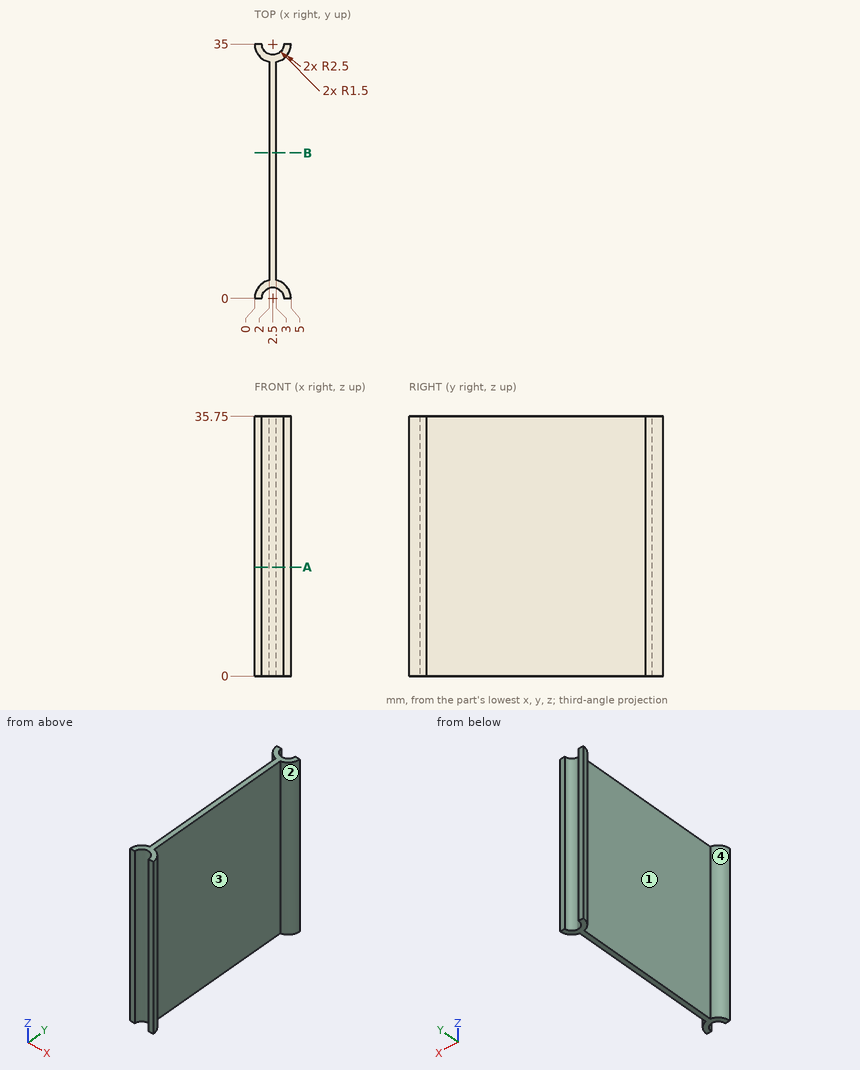
For this review, use the dimensioned drawing (mm, ordinates from the lowest corner) and the shaded views. A direction names the side the tool comes from. Round coordinates to 2 decimals unless told otherwise and drop trailing zeros. Order: outer loops, then holes, each group sorted by start corner. A loop starts at its lowest first (then second) coordinate and runs counter-clockwise, first axis right, second up. Notation, with made-up numbers: M -2.75,-7 L 33.25,-7 A12 cw 33.25,3 Z; hole C -12.75,46.5 d10. An arc over 180 degrees is marked long. Use a Markdown table: item, result. Add a question column.
Item 1: Add section B-B, the plane y = 20. Give the boundary of the cut face in (x, z), then the cut area to 4 significant figures.
Item 2: Insertion check: pin 1 (1.5 mm diameter, centred on x = 1, y = 12, fed in from -Z); pin 2 (3 mm diameter, centred on x = 3, z = 26.5, fed in from +Y); pin 3 (9 mm diameter, centred on y = 23, z = 12.5, fed in from -X). Each pin has a flat end and moves straight along its axis. Give the tip position at first contact, or say it passes through.
Item 3: Mouldability with a two-part tool opening along Y and no side actions: class the marked faces 3 and 4 as released by +Y, released by -Y, zero draft, split by the parting line, or undercut.
Item 4: Add section A-A, the plane z = 15. Give the boundary of the cut face in (x, y), then the cut area to 3 significant figures.
Item 5: To check wall thickness, follow line 1 along X through (y, z) = (7.5, 32); line 2 along Y through (x, z) = (2.6, 23.5); line 3 along Y through (x, z) = (1.8, 2.5). State the ranges of each line that lie inside material, in increasing order.
Item 6: Tool access review of the marked faces 1 and 2: name each direction out of +Z, -Z, +X, -X, +Y, -Y from which nothing blocks a thin tool from reaching the whole face with its end or side.
Geometry results:
| question | item | result |
|---|---|---|
| 1 | outline | M 2,0 L 3,0 L 3,35.75 L 2,35.75 Z |
| 1 | area | 35.75 mm² |
| 2 | pin 1 | passes through |
| 2 | pin 2 | stops at y = 35 |
| 2 | pin 3 | stops at x = 2 |
| 3 | face 3 | undercut |
| 3 | face 4 | undercut |
| 4 | outline | M 0,0 L 1,0 A1.5 cw 4,0 L 5,0 A2.5 ccw 3,2.45 L 3,32.55 A2.5 ccw 5,35 L 4,35 A1.5 cw 1,35 L 0,35 A2.5 ccw 2,32.55 L 2,2.45 A2.5 ccw Z |
| 4 | area | 42.6 mm² |
| 5 | line 1 | x = 2 to 3 |
| 5 | line 2 | y = 1.5 to 33.5 |
| 5 | line 3 | y = 1.33 to 2.4, 32.6 to 33.67 |
| 6 | face 1 | +Z, -Z, -X |
| 6 | face 2 | +Z, -Z, +X |
